Model file for the job. Use its own axes, mm. Face numbers are marked on the shaded views. A direction names the side the tool comes from. Coordinates: 2 decimals unless noted, no trailing zeros. Loops run counter-clockwise (first coordinate to the right, second up) from the corner with the lowest first, then second, coordinate; pieces in that order, holes last. Notation, with made-up numbers: (53, 23.25) - (70, 23.25) arc R20 ccw to (70, 27.25) - close; hole circle Ø6 at (14, 76). An arc over 180 degrees is marked (long way). Write each question's results on one line, items separated by ' | '. Start each with the question number.
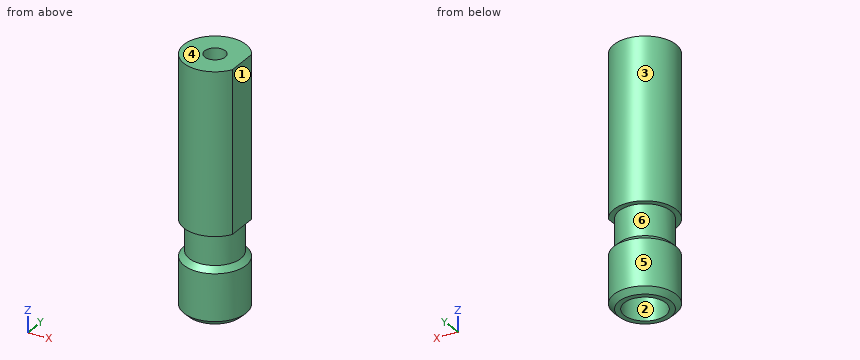
```python
from build123d import *

# Parameters (mm, degrees)
BOSS_EXTRUDE1_DEPTH                                 = 15.5
CBORE_FOR_1_BINDING_HEAD_MACHINE_SCREW1_D           = 2
CBORE_FOR_1_BINDING_HEAD_MACHINE_SCREW1_DEPTH       = 24
CBORE_FOR_1_BINDING_HEAD_MACHINE_SCREW1_CBORE_D     = 4
CBORE_FOR_1_BINDING_HEAD_MACHINE_SCREW1_CBORE_DEPTH = 22
CHAMFER1_SIZE                                       = 0.5


with BuildPart() as part:
    # Sketch1 → Boss-Extrude1 (new body)
    with BuildSketch(Plane(origin=(0, 0, 8.5), x_dir=(-1, 0, 0), z_dir=(0, 0, -1))):
        with BuildLine():
            Line((-2.6, 1.496662955), (-2.6, -1.496662955))
            ThreePointArc((-2.6, -1.496662955), (3, 0), (-2.6, 1.496662955))
        make_face()
    extrude(amount=-BOSS_EXTRUDE1_DEPTH)

    # Sketch2 → Revolve1 (revolve)
    with BuildSketch(Plane.XZ):
        Polygon((2.5, 8.5), (0, 8.5), (0, 0), (3, 0), (3, 5), (2.5, 5.5), align=None)
    revolve(axis=Axis((0, 0, 8.5), (0, 0, -1)))

    # CBORE for #1 Binding Head Machine Screw1
    with Locations(Plane(origin=(0, 0, 0), x_dir=(-1, 0, 0), z_dir=(0, 0, -1))):
        with Locations((0, 0)):
            CounterBoreHole(CBORE_FOR_1_BINDING_HEAD_MACHINE_SCREW1_D / 2, CBORE_FOR_1_BINDING_HEAD_MACHINE_SCREW1_CBORE_D / 2, CBORE_FOR_1_BINDING_HEAD_MACHINE_SCREW1_CBORE_DEPTH, depth=CBORE_FOR_1_BINDING_HEAD_MACHINE_SCREW1_DEPTH)

    # Chamfer1
    chamfer1_edges = [part.edges().sort_by_distance(p)[0] for p in [
        (-3, 0, 0),
    ]]
    chamfer(chamfer1_edges, length=CHAMFER1_SIZE)


solid = part.part
```
Q1. Cut at B-B (x = 0). List the corners of the cut face in (y, z).
Q2. Cut at D-D (z = 15). List the corners of the cut face in (x, y), and give its area (3 significant figures).
Q3. Cut at A-A (y = 0). List the corners of the cut face in (x, z), and give its area (3 significant figures).
Q4. Drill centre lines: L1, parallel to Y at x = 0.15, z = 6.75; L2, parallel to Y at x = 0, z = 23.35; L3, parallel to X at y = -1.75, z = 21. Where is each one in solid material? Low to high. Write a range as from..to.
Q5. Cut at C-C (z = 3). List the corners of the cut face in (x, y).
Q6. Pin check, flat tips, straight feed: pin 1 (1 mm diameter, centred on x = -1.5, z = 18, fed in from +Y); pin 2 (2.5 mm diameter, centred on y = -0.5, z = 18.5, fed in from +X); pin 3 (1.8 mm diameter, centred on x = 0, y = 0, fed in from +Z); pin 4 (1 mm diameter, centred on x = 1, z = 11, fed in from -Y). Stop position of each tip, or through.
Q7. Mould opens along Z. For the marked faces 4, 5 and 6 say: +Z half, -Z half, draft (parallel to the pull), parting line (faces both ways), or undercut.
Q8. Which spindle directions (+Z, -Z, +X, -X, +Y, -Y) get a long thin tool onto all of the face, cutting with end or side? Do the marked faces 1, 2 and 3. Say none if no direction does.
Check result:
1) outline: (-3, 0.5) - (-2.5, 0) - (-2, 0) - (-2, 22) - (-1, 22) - (-1, 24) - (-3, 24) - (-3, 8.5) - (-2.5, 8.5) - (-2.5, 5.5) - (-3, 5) - close; (1, 22) - (2, 22) - (2, 0) - (2.5, 0) - (3, 0.5) - (3, 5) - (2.5, 5.5) - (2.5, 8.5) - (3, 8.5) - (3, 24) - (1, 24) - close
2) outline: (2.6, -1.5) - (2.6, 1.5) arc R3 ccw (long way) to start; hole circle Ø4 at (0, 0) | area: 14.9 mm²
3) outline: (-3, 0.5) - (-2.5, 0) - (-2, 0) - (-2, 22) - (-1, 22) - (-1, 24) - (-3, 24) - (-3, 8.5) - (-2.5, 8.5) - (-2.5, 5.5) - (-3, 5) - close; (1, 22) - (2, 22) - (2, 0) - (2.5, 0) - (3, 0.5) - (3, 5) - (2.5, 5.5) - (2.5, 8.5) - (2.6, 8.5) - (2.6, 24) - (1, 24) - close | area: 42.3 mm²
4) L1: -2.5..-1.99, 1.99..2.5 | L2: -3..-1, 1..3 | L3: -2.44..-0.97, 0.97..2.44
5) outline: circle Ø6 at (0, 0); hole circle Ø4 at (0, 0)
6) pin 1: y = 2.83 | pin 2: x = 2.6 | pin 3: through | pin 4: y = -2.96
7) face 4: +Z half | face 5: draft | face 6: undercut
8) face 1: +Z, +X, +Y, -Y | face 2: -Z | face 3: +Z, -Z
